Autodesk Inventor part; units mm, degrees
ref_plane "YZ Plane" through (0, 0, 0) normal (1, 0, 0) x (0, 1, 0)
ref_plane "XZ Plane" through (0, 0, 0) normal (0, 1, 0) x (-1, 0, 0)
ref_plane "XY Plane" through (0, 0, 0) normal (0, 0, 1) x (1, 0, 0)
sketch "Эскиз1" plane through (0, 0, 0) normal (0, 1, 0) x (-1, 0, 0)
  circle A0 centre (0, 0) radius 2.45
  circle A1 centre (0, 0) radius 3.75
  dimension "d0" = 4.9
  dimension "d1" = 7.5
extrude "Выдавливание1" add sketch "Эскиз1" along normal blind 6
sketch "Эскиз2" plane through (0, 0, 0) normal (1, 0, 0) x (0, 1, 0)
  circle A0 centre (3, 0) radius 1.25
  line L0 (0, -3.75) -> (0, 3.75)
  circle A1 centre (3, 0) radius 3
  circle A2 centre (3, 7.071) radius 1.25
  arc A3 (6, 7.071) -> (0, 7.071) centre (3, 7.071) ccw
  line L1 (3, 0) -> (3, 7.071) construction
  line L2 (6, 0) -> (6, 7.071)
  line L3 (0, 7.071) -> (0, 0)
  point P0 (0, 0)
  dimension "d7" = 6
  dimension "d4" = 2.5
  dimension "d12" = 2.5
  dimension "d13" = 6
  dimension "d14" = 7.071
extrude "Выдавливание3" add sketch "Эскиз2" along normal mid plane 7.5 contours A1
extrude "Выдавливание5" add sketch "Эскиз2" along normal blind 1.85 and the other way blind 3.75 contours L0 L3 A3 L2 A1
extrude "Выдавливание2" add sketch "Эскиз2" along normal mid plane 11 contours A0
extrude "Выдавливание4" cut sketch "Эскиз1" along normal blind 6 contours A0
extrude "Выдавливание7" add sketch "Эскиз2" along normal blind 3.6 and the other way blind 5.5 contours A2
sketch "Эскиз3" plane through (1.85, 0, 0) normal (1, 0, 0) x (0, 0, -1)
  circle A0 centre (-7.071, 3) radius 1.25
  arc A1 (-7.071, 6) -> (-7.071, 0) centre (-7.071, 3) ccw
  arc A2 (-7.071, 0) -> (-7.071, 6) centre (-7.071, 3) ccw
  line L0 (-7.071, 0) -> (-3.2619, 0)
  line L1 (0, 0) -> (-3.2619, 0)
  line L2 (3.75, 0) -> (0, 0)
  line L3 (-4.9497, 5.1213) -> (0, 0)
  point P0 (-4.8786, 5.0478)
extrude "Выдавливание8" cut sketch "Эскиз3" along normal blind 3.75
properties part number "Кулак"
For this review, take the finished solid that the model builds, in its own axes (mm). A direction names the side the tool comes from. Round coordinates to 2 decimals unless told otherwise and drop trailing zeros. Order: outer loops, then holes, each group sorted by start corner. A loop starts at its lowest first (then second) coordinate and runs counter-clockwise, first axis right, second up. Notation, with made-up numbers: (3, 33.5) -> (33, 33.5) arc R33 ccw to (33, 63.5) -> close; hole circle Ø10 at (-39.75, 20). An arc over 180 degrees is marked (long way). Write item = value, one per line. Start each with the question number.
1) To check wall thickness, follow line 1 (X direction, y = 3.1, z = 0); line 2 (X direction, y = 3, z = -1); line 3 (Z direction, x = 0, y = 4.3). State the ranges of each line that lie inside material, in increasing order. Write a range as from..to.
2) Take a section at A-A on x = 0. State the section outline as (y, z) points, plus the area to 3 significant figures.
3) Take a section at D-D on x = 4.5. State the section outline as (y, z) points.
4) Insertion check: pin 1 (2 mm diameter, centred on y = 0.5, z = 8.5, fed in from -X); pin 2 (3 mm diameter, centred on y = 4.5, z = 6, fed in from +X). Each pin has a flat end and moves straight along its axis. Give the tip position at first contact, or say it passes through.
5) The part is to be moulded in two halves that separate along Z. For faces 6 (the face through (-3.75, 3, 4)), 7 (the face through (3, 3, -3)), 8 (the face through (-0.99, 2.93, 10.07)), 9 (the face through (5.5, 3, 0)), say which applies: +Z half, -Z half, draft (parallel to the pull), parting line (faces both ways), or undercut.
6) Take a section at C-C on z = 2.75. State the section outline as (x, y) points, plus the area to 3 significant figures.
7) Take a section at B-B on y = 2.75. State the section outline as (x, z) points.
8) Tool access review of faces 1 (the face through (2.6, 5.1, 2.7)), 2 (the face through (-4.613, 3.577, 5.962)), 3 (the face through (-3, 3, -3)), 4 (the face through (2.79, 1.71, 1.65)), 5 (the face through (4.61, 4.19, -0.38)): name each direction out of +Z, -Z, +X, -X, +Y, -Y from which nothing blocks a thin tool from reaching the whole face with its end or side.
Verdict:
q1.line_1 = -5.5..-2.45, 2.45..5.5
q1.line_2 = -5.5..-2.24, 2.24..5.5
q1.line_3 = -3.75..-2.45, 2.45..9.77
q2.outline = (0, -3.75) -> (6, -3.75) -> (6, -2.45) -> (0, -2.45) -> close; (0, 2.45) -> (6, 2.45) -> (6, 7.07) arc R3 ccw to (0, 7.07) -> close
q2.area = 49.7 mm2
q3.outline = circle Ø2.5 at (3, 0)
q4.pin_1 = -3.75
q4.pin_2 = 1.85
q5.face_6 = undercut
q5.face_7 = -Z half
q5.face_8 = +Z half
q5.face_9 = draft
q6.outline = (-3.75, 0) -> (1.85, 0) -> (1.85, 2.85) -> (3.75, 2.85) -> (3.75, 4.2) -> (2.55, 4.2) -> (2.55, 6) -> (-3.75, 6) -> close
q6.area = 37.4 mm2
q7.outline = (-5.5, -1.22) -> (-3.75, -1.22) -> (-3.75, -2.99) -> (-2.26, -2.99) arc R3.75 ccw to (2.26, -2.99) -> (3.75, -2.99) -> (3.75, -1.22) -> (5.5, -1.22) -> (5.5, 1.22) -> (3.75, 1.22) -> (3.75, 2.66) -> (1.85, 2.66) -> (1.85, 10.06) -> (-3.75, 10.06) -> (-3.75, 8.3) -> (-5.5, 8.3) -> (-5.5, 5.85) -> (-3.75, 5.85) -> (-3.75, 1.22) -> (-5.5, 1.22) -> close; hole circle Ø4.9 at (0, 0)
q8.face_1 = +Z, +X, +Y
q8.face_2 = -X
q8.face_3 = -Z, -X
q8.face_4 = +Z, +X, -Y
q8.face_5 = +X
